Here's how the part is built. I have some questions about the finished solid (model axes, mm). Face numbers are marked on the shaded views. Give positions to 0.01 mm unless a question says otherwise; leave off trailing zeros. Order: outer loops, then holes, each group sorted by start corner. A loop starts at its lowest first (then second) coordinate and runs counter-clockwise, first axis right, second up. Notation, with made-up numbers: M 58.5,-21 L 114.5,-21 A26 cw 114.5,15 Z; hole C 27,39.25 d8. An arc over 180 degrees is marked long. Use one line per item in the form item = value.
from build123d import *

# Parameters (mm, degrees)
BOSS_EXTRUDE5_DEPTH         = 22.85
BOSS_EXTRUDE5_DEPTH_BACK    = 0.00254
SKETCH1_R                   = 46.45
SKETCH1_12_R                = 44.45
CUT_EXTRUDE13_DEPTH         = 70.550898628
F_3_16_0_1875_DOWEL_HOLE1_D = 4.7625
F_3_16_0_1875_DOWEL_HOLE3_D = 4.7625
F_3_16_0_1875_DOWEL_HOLE4_D = 4.7625
F_3_16_0_1875_DOWEL_HOLE5_D = 4.7625
SKETCH1_21_R                = 44.45
SKETCH1_21_R_2              = 42.45
BOSS_EXTRUDE16_DEPTH        = 16.5
BOSS_EXTRUDE15_DEPTH        = 16.5
CUT_EXTRUDE21_DEPTH         = 70.550898628
CUT_EXTRUDE21_DEPTH_BACK    = 4
SKETCH24_4_R                = 2.286
SKETCH25_R                  = 42.45
BOSS_EXTRUDE17_DEPTH        = 2
CUT_EXTRUDE22_DEPTH         = 70.550898628
CUT_EXTRUDE22_DEPTH_BACK    = 70.550898628
SKETCH21_R                  = 1.3
SKETCH21_R_2                = 1.3000014
SKETCH21_W                  = 11.5
SKETCH21_H                  = 21
SKETCH26_R                  = 2.38125
CUT_EXTRUDE23_DEPTH         = 3


with BuildPart() as part:
    # Sketch1 → Boss-Extrude5 (new, two sides: drawn at the far end of the back side and taken through both)
    with BuildSketch(Plane.XY.offset(-BOSS_EXTRUDE5_DEPTH_BACK)):
        Circle(SKETCH1_R)
    extrude(amount=BOSS_EXTRUDE5_DEPTH + BOSS_EXTRUDE5_DEPTH_BACK)

    # Sketch1_12 → Cut-Extrude13 (cut, through all)
    with BuildSketch(Plane.XY):
        with Locations(Location((0, 0, 0), (0, 0, 180))):
            Circle(SKETCH1_12_R)
    extrude(amount=CUT_EXTRUDE13_DEPTH, mode=Mode.SUBTRACT)

    # 3_16 _0.1875_ Dowel Hole1 (through all)
    with Locations(Plane.XY):
        with Locations((-29.21, 17.000000036)):
            Hole(F_3_16_0_1875_DOWEL_HOLE1_D / 2)

    # 3_16 _0.1875_ Dowel Hole3 (through all)
    with Locations(Plane.XY):
        with Locations((-29.21, -16.999999964)):
            Hole(F_3_16_0_1875_DOWEL_HOLE3_D / 2)

    # 3_16 _0.1875_ Dowel Hole4 (through all)
    with Locations(Plane.XY):
        with Locations((29.21, -16.999999964)):
            Hole(F_3_16_0_1875_DOWEL_HOLE4_D / 2)

    # 3_16 _0.1875_ Dowel Hole5 (through all)
    with Locations(Plane.XY):
        with Locations((29.21, 17.000000036)):
            Hole(F_3_16_0_1875_DOWEL_HOLE5_D / 2)

    # Sketch1_21 → Boss-Extrude16 (add)
    with BuildSketch(Plane.XY):
        with Locations(Location((0, 0, 0), (0, 0, 180))):
            Circle(SKETCH1_21_R)
        Circle(SKETCH1_21_R_2, mode=Mode.SUBTRACT)
    extrude(amount=BOSS_EXTRUDE16_DEPTH)

    # Sketch24 → Boss-Extrude15 (add)
    with BuildSketch(Plane.XY):
        with BuildLine():
            Line((31.373699445, 13.282255292), (40.400761439, 18.535937395))
            ThreePointArc((40.400761439, 18.535937395), (38.421298232, 22.351875586), (36.082481048, 25.958756932))
            Line((36.082481048, 25.958756932), (27.054115803, 20.704316346))
            ThreePointArc((27.054115803, 20.704316346), (25.50568369, 14.844115839), (31.365884197, 13.295683726))
            Line((31.365884197, 13.295683726), (31.373699445, 13.282255292))
        make_face()
        with BuildLine():
            ThreePointArc((36.120106654, -25.906377502), (38.433582829, -22.330745866), (40.394249477, -18.550124237))
            Line((40.394249477, -18.550124237), (31.365884191, -13.29568365))
            ThreePointArc((31.365884191, -13.29568365), (25.333011542, -15.172773516), (27.725141272, -21.020570888))
            Line((27.725141272, -21.020570888), (36.120106654, -25.906377502))
        make_face()
        with BuildLine():
            Line((-27.054115803, 20.704316346), (-36.082481048, 25.958756932))
            ThreePointArc((-36.082481048, 25.958756932), (-38.41737284, 22.358621694), (-40.394249443, 18.550124311))
            Line((-40.394249443, 18.550124311), (-31.365884197, 13.295683726))
            ThreePointArc((-31.365884197, 13.295683726), (-25.50568369, 14.844115839), (-27.054115803, 20.704316346))
        make_face()
        with BuildLine():
            ThreePointArc((-40.394249477, -18.550124237), (-38.417372882, -22.358621623), (-36.082481096, -25.958756865))
            Line((-36.082481096, -25.958756865), (-27.054115809, -20.704316278))
            ThreePointArc((-27.054115809, -20.704316278), (-25.505683686, -14.844115773), (-31.365884191, -13.29568365))
            Line((-31.365884191, -13.29568365), (-40.394249477, -18.550124237))
        make_face()
    extrude(amount=BOSS_EXTRUDE15_DEPTH)

    # Sketch24_4 → Cut-Extrude21 (cut, two sides: drawn at the far end of the back side and taken through both)
    with BuildSketch(Plane.XY.offset(-CUT_EXTRUDE21_DEPTH_BACK)):
        with Locations((29.21, 17.000000036)):
            Circle(SKETCH24_4_R)
        with Locations((29.21, -16.999999964)):
            Circle(SKETCH24_4_R)
        with Locations((-29.21, 17.000000036)):
            Circle(SKETCH24_4_R)
        with Locations((-29.21, -16.999999964)):
            Circle(SKETCH24_4_R)
    extrude(amount=CUT_EXTRUDE21_DEPTH + CUT_EXTRUDE21_DEPTH_BACK, mode=Mode.SUBTRACT)

    # Sketch25 → Boss-Extrude17 (add)
    with BuildSketch(Plane.XY):
        Circle(SKETCH25_R)
    extrude(amount=BOSS_EXTRUDE17_DEPTH)

    # Sketch21 → Cut-Extrude22 (cut, two sides: drawn at the far end of the back side and taken through both)
    with BuildSketch(Plane.XY.offset(-CUT_EXTRUDE22_DEPTH_BACK)):
        with Locations(Location((-5.5, 9, 0), (0, 0, 180))):
            Circle(SKETCH21_R)
        with Locations(Location((5.5, 9, 0), (0, 0, 180))):
            Circle(SKETCH21_R)
        with Locations(Location((5.5, -9, 0), (0, 0, 180))):
            Circle(SKETCH21_R)
        with Locations(Location((-5.5, -9, 0), (0, 0, 180))):
            Circle(SKETCH21_R_2)
        with Locations((-14.25, 0)):
            Rectangle(SKETCH21_W, SKETCH21_H)
    extrude(amount=CUT_EXTRUDE22_DEPTH + CUT_EXTRUDE22_DEPTH_BACK, mode=Mode.SUBTRACT)

    # Sketch26 → Cut-Extrude23 (cut)
    with BuildSketch(Plane(origin=(0, 0, -0.00254), x_dir=(-1, 0, 0), z_dir=(0, 0, -1))):
        with Locations(Location((29.21, -16.999999964, 0), (0, 0, 180))):
            Circle(SKETCH26_R)
        with Locations(Location((29.21, 17.000000036, 0), (0, 0, 180))):
            Circle(SKETCH26_R)
        with Locations(Location((-29.21, 17.000000036, 0), (0, 0, 180))):
            Circle(SKETCH26_R)
        with Locations(Location((-29.21, -16.999999964, 0), (0, 0, 180))):
            Circle(SKETCH26_R)
    extrude(amount=-CUT_EXTRUDE23_DEPTH, mode=Mode.SUBTRACT)


solid = part.part
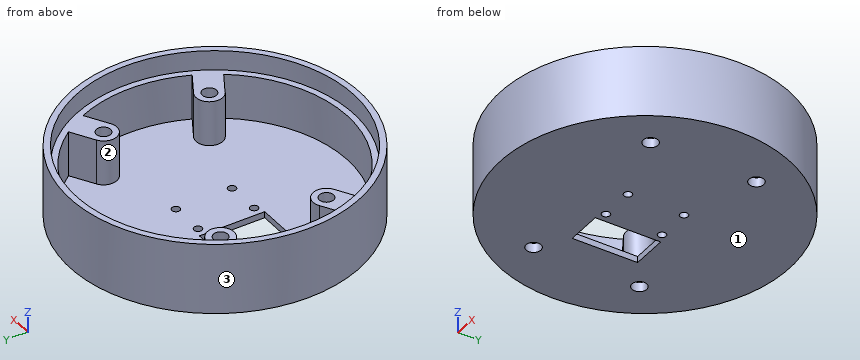
Q1. I need wall thicknesses on L1, parallel to Y at x = 30.5, z = 12.25; L2, parallel to Y at x = 30, z = 5; L3, parallel to Y at x = 0, z = 21. Which ranges of each line are inside material? Lowest first, please.
Found:
L1 = -35.03 to -29.53, -22.64 to -18.89, -15.11 to -12.91, 12.91 to 15.11, 18.89 to 22.71, 29.53 to 35.03
L2 = -35.46 to -30.03, -22.34 to -19.15, -14.85 to -12.79, 12.79 to 14.85, 19.15 to 22.42, 30.03 to 35.46
L3 = -46.45 to -44.45, 44.45 to 46.45
Q2. I want a section at A-A on x = 5.5. Write out the boundary of the cut face in (y, z), then the cut area to 3 significant figures.
Found:
outline = M -46.12,0 L -10.3,0 L -10.3,2 L -42.09,2 L -42.09,16.5 L -44.11,16.5 L -44.11,22.85 L -46.12,22.85 Z; M -7.7,0 L 7.7,0 L 7.7,2 L -7.7,2 Z; M 10.3,0 L 46.12,0 L 46.12,22.85 L 44.11,22.85 L 44.11,16.5 L 42.09,16.5 L 42.09,2 L 10.3,2 Z
area = 317 mm²
Q3. I want a section at B-B on y = 9. Write out the boundary of the cut face in (x, z), then the cut area to 3 significant figures.
Found:
outline = M -45.57,0 L -20,0 L -20,2 L -41.48,2 L -41.48,16.5 L -43.53,16.5 L -43.53,22.85 L -45.57,22.85 Z; M -8.5,0 L -6.8,0 L -6.8,2 L -8.5,2 Z; M -4.2,0 L 4.2,0 L 4.2,2 L -4.2,2 Z; M 6.8,0 L 45.57,0 L 45.57,22.85 L 43.53,22.85 L 43.53,16.5 L 41.48,16.5 L 41.48,2 L 6.8,2 Z
area = 293 mm²
Q4. I'm going to push flat-ended pins straight in: pin 1 Ø5.5 at (x, y) = (-29.21, 17) entering from +Z; pin 2 Ø2 at (x, z) = (-12.5, 1.5) entering from +Y; pin 3 Ø0.6 at (y, z) = (-4, 1) entering from -X. Where does each tip first touch, or does it pass through?
Found:
pin_1 = 16.5
pin_2 = 45
pin_3 = -46.3
Q5. I want a section at D-D on x = 23.5. Write out the boundary of the cut face in (y, z), then the cut area to 3 significant figures.
Found:
outline = M -40.07,0 L 40.07,0 L 40.07,22.85 L 37.73,22.85 L 37.73,16.5 L 35.35,16.5 L 35.35,2 L -35.35,2 L -35.35,16.5 L -37.73,16.5 L -37.73,22.85 L -40.07,22.85 Z
area = 327 mm²
Q6. Thinking about a two-plate mould opening in X: for the marked faces 1, 2 and 3, which applies, +X half, -X half, draft (parallel to the pull), parting line (faces both ways), or undercut?
Found:
face_1 = draft
face_2 = undercut
face_3 = parting line
Q7. I want a section at C-C on z = 20.25. Write out the boundary of the cut face in (x, y).
Found:
outline = C 0,0 d92.9; hole C 0,0 d88.9
